```python
from build123d import *

# Parameters (mm, degrees)
BOSS_EXTRUDE1_DEPTH = 5


with BuildPart() as part:
    # Sketch1 → Boss-Extrude1 (new body)
    with BuildSketch(Plane(origin=(0, 0, 0), x_dir=(1, 0, 0), z_dir=(0, 1, 0))):
        with BuildLine():
            Line((115, 160.4), (110, 160.4))
            Line((110, 160.4), (110, 182.966371269))
            ThreePointArc((110, 182.966371269), (0, 191.663253961), (-110, 182.966371269))
            Line((-110, 182.966371269), (-110, 160.4))
            Line((-110, 160.4), (-115, 160.4))
            Line((-115, 160.4), (-115, 182.15221115))
            ThreePointArc((-115, 182.15221115), (-142.899993603, 176.922031233), (-170.565, 170.565))
            ThreePointArc((-170.565, 170.565), (-176.922031233, 142.899993603), (-182.15221115, 115))
            Line((-182.15221115, 115), (-160.4, 115))
            Line((-160.4, 115), (-160.4, 110))
            Line((-160.4, 110), (-182.966371269, 110))
            ThreePointArc((-182.966371269, 110), (-191.663253961, 0), (-182.966371269, -110))
            Line((-182.966371269, -110), (-160.4, -110))
            Line((-160.4, -110), (-160.4, -115))
            Line((-160.4, -115), (-182.15221115, -115))
            ThreePointArc((-182.15221115, -115), (-176.922031233, -142.899993603), (-170.565, -170.565))
            ThreePointArc((-170.565, -170.565), (-142.899993603, -176.922031233), (-115, -182.15221115))
            Line((-115, -182.15221115), (-115, -160.4))
            Line((-115, -160.4), (-110, -160.4))
            Line((-110, -160.4), (-110, -182.966371269))
            ThreePointArc((-110, -182.966371269), (0, -191.663253961), (110, -182.966371269))
            Line((110, -182.966371269), (110, -160.4))
            Line((110, -160.4), (115, -160.4))
            Line((115, -160.4), (115, -182.15221115))
            ThreePointArc((115, -182.15221115), (142.899993603, -176.922031233), (170.565, -170.565))
            ThreePointArc((170.565, -170.565), (176.922031233, -142.899993603), (182.15221115, -115))
            Line((182.15221115, -115), (160.4, -115))
            Line((160.4, -115), (160.4, -110))
            Line((160.4, -110), (182.966371269, -110))
            ThreePointArc((182.966371269, -110), (191.663253961, 0), (182.966371269, 110))
            Line((182.966371269, 110), (160.4, 110))
            Line((160.4, 110), (160.4, 115))
            Line((160.4, 115), (182.15221115, 115))
            ThreePointArc((182.15221115, 115), (176.922031233, 142.899993603), (170.565, 170.565))
            ThreePointArc((170.565, 170.565), (142.899993603, 176.922031233), (115, 182.15221115))
            Line((115, 182.15221115), (115, 160.4))
        make_face()
    extrude(amount=BOSS_EXTRUDE1_DEPTH)


solid = part.part
```
Model file for the job. Use its own axes, mm. Give positions to 0.01 mm unless a question says otherwise; leave off trailing zeros. Order: outer loops, then holes, each group sorted by start corner. A loop starts at its lowest first (then second) coordinate and runs counter-clockwise, first axis right, second up.
1) Pin check, flat tips, straight feed: pin 1 (1.5 mm diameter, centred on y = 3, z = -113, fed in from -X); pin 2 (1.5 mm diameter, centred on x = 169, y = 2.5, fed in from -Z); pin 3 (2.5 mm diameter, centred on x = -171, y = 3.5, fed in from -Z). Stop position of each tip, or through.
2) Saw through at B-B, the plane x = -141. Write the cut outline in (y, z), then the cut area to 3 significant figures.
3) Wall check: probe 1 along Z at (x, y) = (160.5, 4.35); probe 2 along X at (y, z) = (1.85, 59.5); probe 3 along Z at (x, y) = (148, 4.8). Give the ranges that are in metal, low to high.
4) Saw through at A-A, the plane z = -66.5. Write the cut outline in (x, y).
Computed:
1. pin 1: stops at x = -160.4
1. pin 2: stops at z = -171.14
1. pin 3: stops at z = -170.77
2. outline: (0, -177.32) - (5, -177.32) - (5, 177.32) - (0, 177.32) - close
2. area: 1,770 mm2
3. probe 1: z = -173.01 to -115, -110 to 110, 115 to 173.01
3. probe 2: x = -189.13 to 189.13
3. probe 3: z = -175.84 to 175.84
4. outline: (-188.5, 0) - (188.5, 0) - (188.5, 5) - (-188.5, 5) - close
